Can you work these out from the model? Positions are in its coordinate system, mm. A direction names the side the tool comes from. Coordinates: 2 decimals unless noted, no trailing zeros. Loops run counter-clockwise (first coordinate to the right, second up) from the corner with the lowest first, then second, coordinate; pieces in that order, holes last.
```python
from build123d import *

# Parameters (mm, degrees)
PAD_DEPTH    = 6
SKETCH001_R  = 1.7
POCKET_DEPTH = 98.087915


with BuildPart() as part:
    # Sketch → Pad (new body)
    with BuildSketch(Plane.XY):
        Polygon((-20, -5), (-20, 5), (-10, 5), (-10, 11), (10, 11), (10, 5), (20, 5), (20, -5), (10, -5), (10, -11), (-10, -11), (-10, -5), align=None)
    extrude(amount=PAD_DEPTH)

    # Sketch001 (on Face14 of Pad) → Pocket (cut, through all)
    with BuildSketch(Plane.XY.offset(6)):
        with Locations((0, 8)):
            Circle(SKETCH001_R)
    pocket = extrude(amount=-POCKET_DEPTH, mode=Mode.SUBTRACT)

    # Mirrored: Pocket across Sketch001 H_Axis
    add(pocket.mirror(Plane(origin=(0, 0, 6), x_dir=(0, 0, 1), z_dir=(0, 1, 0))), mode=Mode.SUBTRACT)


solid = part.part
```
(1) I'm going to push flat-ended pins straight in: pin 1 (3 mm diameter, centred on y = -8.5, z = 1.5, fed in from +X); pin 2 (3 mm diameter, centred on y = -9, z = 4, fed in from -X); pin 3 (1.8 mm diameter, centred on x = 12.5, z = 2, fed in from +Y). Where does each tip first touch, or does it pass through?
Check values:
pin 1: stops at x = 10
pin 2: stops at x = -10
pin 3: stops at y = 5
(2) If I drill on probe 1 along Y at (x, z) = (0, 3.45); probe 2 along X at (y, z) = (-8, 3.1); probe 3 along Y at (x, z) = (13, 1), over which ranges is the centre line in solid material (lowest first)?
Check values:
probe 1: y = -11 to -9.7, -6.3 to 6.3, 9.7 to 11
probe 2: x = -10 to -1.7, 1.7 to 10
probe 3: y = -5 to 5
(3) I want a section at A-A on x = 0. Write out the boundary of the cut face in (y, z), then the cut area to 3 significant figures.
Check values:
outline: (-11, 0) - (-9.7, 0) - (-9.7, 6) - (-11, 6) - close; (-6.3, 0) - (6.3, 0) - (6.3, 6) - (-6.3, 6) - close; (9.7, 0) - (11, 0) - (11, 6) - (9.7, 6) - close
area: 91.2 mm2
(4) I want a section at B-B on y = 8. Write out the boundary of the cut face in (x, z), then the cut area to 3 significant figures.
Check values:
outline: (-10, 0) - (-1.7, 0) - (-1.7, 6) - (-10, 6) - close; (1.7, 0) - (10, 0) - (10, 6) - (1.7, 6) - close
area: 99.6 mm2
(5) I want a section at C-C on z = 4.85. Write out the boundary of the cut face in (x, y).
Check values:
outline: (-20, -5) - (-10, -5) - (-10, -11) - (10, -11) - (10, -5) - (20, -5) - (20, 5) - (10, 5) - (10, 11) - (-10, 11) - (-10, 5) - (-20, 5) - close; hole circle Ø3.4 at (0, -8); hole circle Ø3.4 at (0, 8)
(6) Which directions (+Z, -Z, +X, -X, +Y, -Y) give clear straight access to the entire face, cutting with the end or side of a thin tool? Please do faces 1 (the flat face through (15, -5, 3)), 2 (the flat face through (-10, 8, 3)), 3 (the flat face through (20, 0, 3)), 4 (the flat face through (-10, -8, 3)), 5 (the flat face through (10, 8, 3)).
Check values:
face 1: +Z, -Z, +X, -Y
face 2: +Z, -Z, -X, +Y
face 3: +Z, -Z, +X, +Y, -Y
face 4: +Z, -Z, -X, -Y
face 5: +Z, -Z, +X, +Y
(7) I want a section at D-D on x = 13. Write out the boundary of the cut face in (y, z).
Check values:
outline: (-5, 0) - (5, 0) - (5, 6) - (-5, 6) - close
